Study the drawing (mm; zero at the part's minimum x, y, z) and answer. Coordinates: 2 decimals unless noted, no trailing zeros. Order: outer loops, then holes, each group sorted by start corner. A loop starts at its lowest first (then second) coordinate and runs counter-clockwise, first axis right, second up. Notation, with made-up numbers: M 21,-16.5 L 73,-16.5 A11 cw 73,-7.5 Z; hole C 65,4.5 d2. An arc over 180 degrees is marked long. Use a Markdown table: item, result. Add a question column.
1) Find section A-A on y = 14.5. Write down the section's boundary in (x, z), plus the area to 3 significant figures.
2) Find section C-C on z = 0.75. Write down the section's boundary in (x, y).
3) The mould has two halves that part along Y. Classify the marked faces 1, 2 and 3: released by +Y, released by -Y, zero draft, split by the parting line, or undercut.
4) This flat-tipped pin is pushed along its axis until it touches: pin 1 Ø1.9 at (x, y) = (15.01, 15.09) entering from -Z. Where does it stop, or does it pass through?
5) Find the intervals of material crossed by probe 1 along X at (y, z) = (2.5, 1.15) (1 decimal); probe 2 along X at (y, z) = (3, 1.45), in increasing order. Write a range as [from, to].
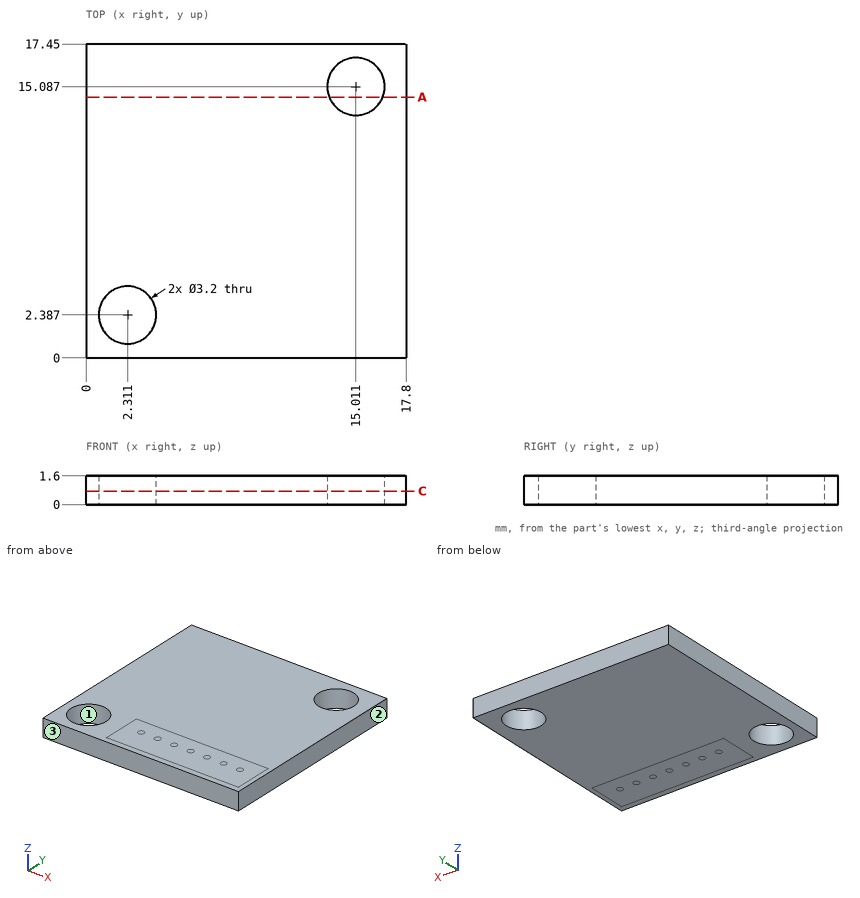
Check result:
| question | item | result |
|---|---|---|
| 1 | outline | M 0,0 L 13.52,0 L 13.52,1.6 L 0,1.6 Z; M 16.5,0 L 17.8,0 L 17.8,1.6 L 16.5,1.6 Z |
| 1 | area | 23.7 mm2 |
| 2 | outline | M 0,0 L 17.8,0 L 17.8,17.45 L 0,17.45 Z; hole C 2.31,2.39 d3.2; hole C 15.01,15.09 d3.2 |
| 3 | face 1 | undercut |
| 3 | face 2 | zero draft |
| 3 | face 3 | released by -Y |
| 4 | pin 1 | passes through |
| 5 | probe 1 | x = [0, 0.7], [3.9, 17.8] |
| 5 | probe 2 | x = [0, 0.83], [3.79, 17.8] |
